Check sheet for the drawn part. Datum: minimum x, y, z corner. Units: mm. Give positions to 0.01 mm unless a question says otherwise; leave off trailing zeros. Write each loop counter-clockwise with the first axis right and the second up, starting at its lowest first coordinate (ties: lowest second). Pieces come first, ordered by that corner, then holes.
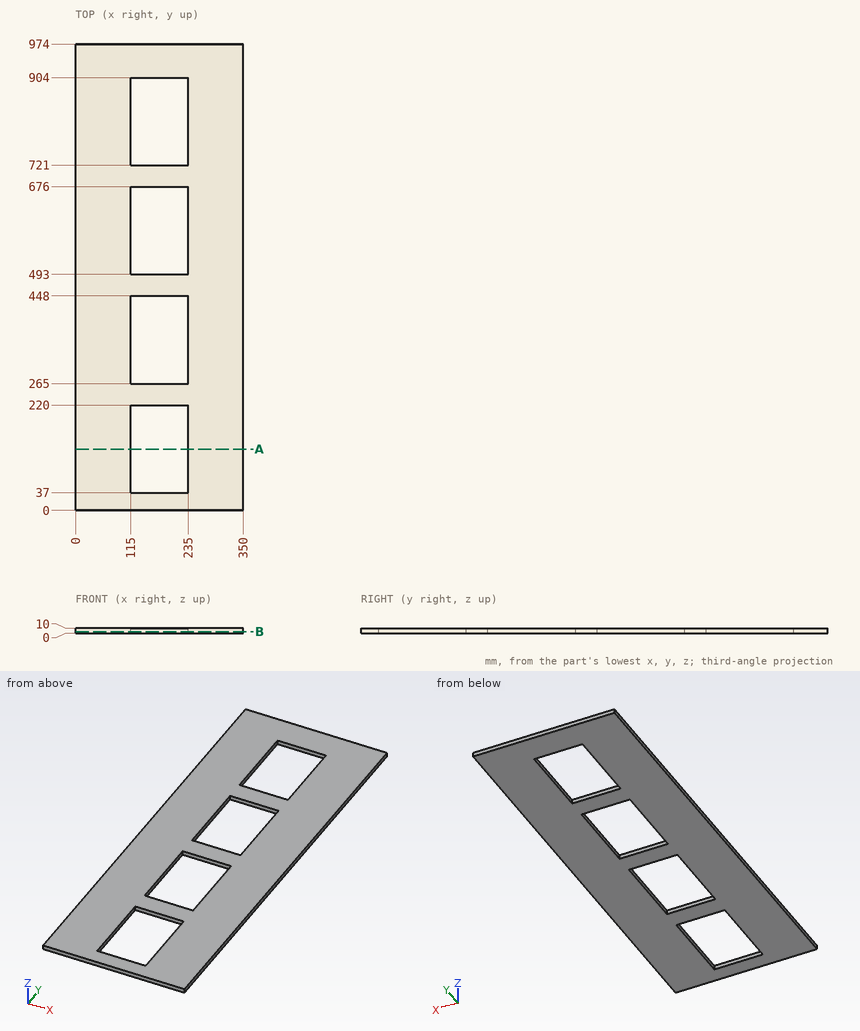
1) Sectioned sample at A-A on y = 128. Record the boundary of the cut face in (x, z), then the cut area to 3 significant figures.
2) Sectioned sample at B-B on z = 3.5. Record the boundary of the cut face in (x, y), then the cut area to 3 significant figures.
3) Scan lines: L1, parallel to Y at x = 146, z = 7.5; L2, parallel to X at y = 298, z = 7.5. Record each from-to range of solid material in increasing order.
Answers below:
1. outline: (0, 0) - (115, 0) - (115, 10) - (0, 10) - close; (235, 0) - (350, 0) - (350, 10) - (235, 10) - close
1. area: 2,300 mm2
2. outline: (0, 0) - (350, 0) - (350, 974) - (0, 974) - close; hole (115, 37) - (235, 37) - (235, 220) - (115, 220) - close; hole (115, 265) - (235, 265) - (235, 448) - (115, 448) - close; hole (115, 493) - (235, 493) - (235, 676) - (115, 676) - close; hole (115, 721) - (235, 721) - (235, 904) - (115, 904) - close
2. area: 253,000 mm2
3. L1: y = 0 to 37, 220 to 265, 448 to 493, 676 to 721, 904 to 974
3. L2: x = 0 to 115, 235 to 350
